The figure shows three views and two pictorial views of one solid part (mm, origin at its lowest corner). Answer the questions. A direction names the side the tool comes from. Give positions to 0.01 mm unless a question says otherwise; leave off trailing zeros. Write each loop counter-clockwise with the first axis right and the second up, starting at its lowest first coordinate (ties: lowest second). Pieces come first, ordered by that corner, then holes. Notation, with made-up numbers: (-16, 0.25) -> (18, 0.25) arc R9 ccw to (18, 5.25) -> close; hole circle Ø2 at (-12, 35). An arc over 180 degrees is marked (long way). Write each question's results on one line, items separated by ' | '. Start each with the question number.
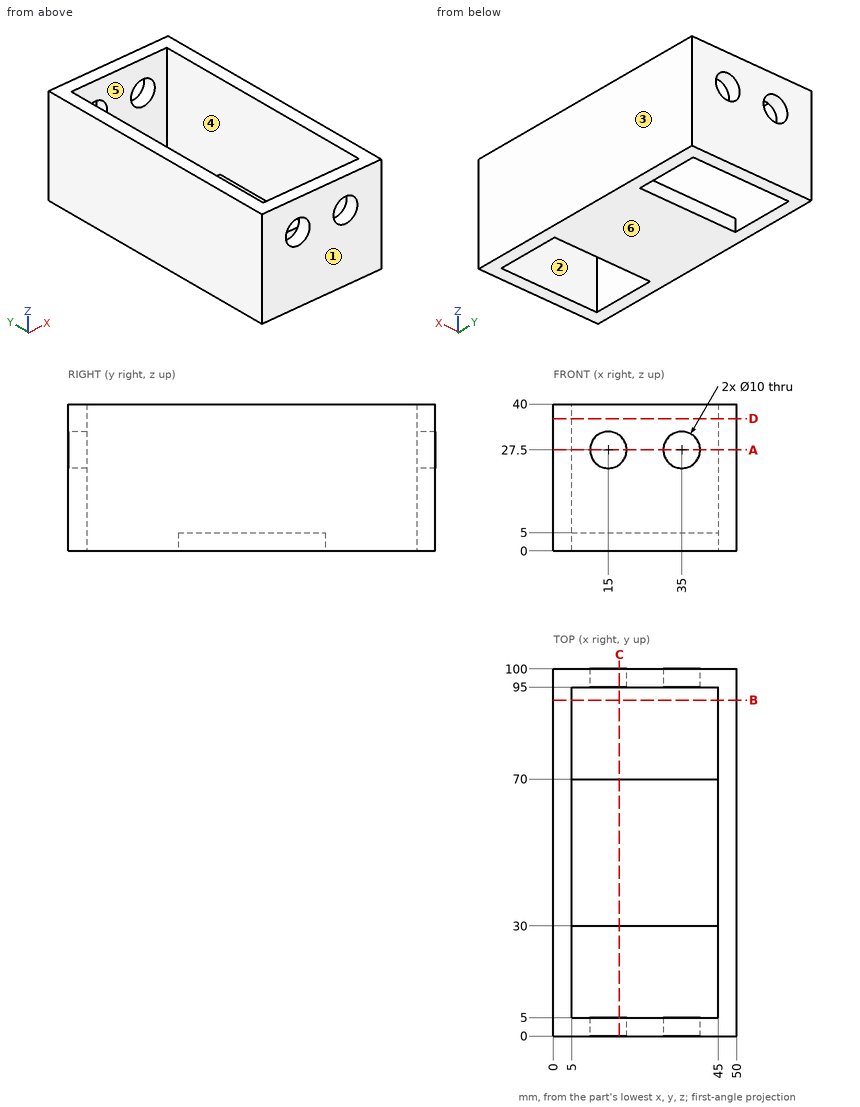
1. Consider probe 1 along Y at (x, z) = (17, 38.5); probe 2 along Z at (x, y) = (15, 97.7); probe 3 along X at (y, z) = (36, 9.5). Determine where each line is inside the solid, lowest interval first. Write a range as [from, to].
2. The mould has two halves that part along Y. Classify the marked faces 1, 2 and 3: pulls with the +Y half, pulls with the -Y half, needs draft (parallel to the pull), parting line crosses it, or undercut.
3. Section B-B (y = 91.5) is taken. Write down the section's boundary in (x, z), then the cut area to 3 significant figures.
4. Section A-A (z = 27.5) is taken. Write down the section's boundary in (x, y).
5. A tool of negligible diameter and unlimited length cuts with its end or side. For the marked faces 4, 5 and 6, from which of +Z, -Z, +X, -X, +Y, -Y can it reach the whole face along a straight path? Write none if from no direction.
6. Section D-D (z = 36) is taken. Write down the section's boundary in (x, y).
7. Section C-C (x = 18) is taken. Write down the section's boundary in (y, z), then the cut area to 3 significant figures.
8. Each of these flat-tipped pins is pushed along its axis until it touches: pin 1 Ø9 at (x, z) = (15, 27.5) entering from +Y; pin 2 Ø20 at (x, y) = (24.5, 46) entering from +Z. Where does it stop, or does it pass through?
Results:
1) probe 1: y = [0, 5], [95, 100] | probe 2: z = [0, 22.5], [32.5, 40] | probe 3: x = [0, 5], [45, 50]
2) face 1: pulls with the -Y half | face 2: undercut | face 3: needs draft
3) outline: (0, 0) -> (5, 0) -> (5, 40) -> (0, 40) -> close; (45, 0) -> (50, 0) -> (50, 40) -> (45, 40) -> close | area: 400 mm²
4) outline: (0, 0) -> (10, 0) -> (10, 5) -> (5, 5) -> (5, 95) -> (10, 95) -> (10, 100) -> (0, 100) -> close; (20, 0) -> (30, 0) -> (30, 5) -> (20, 5) -> close; (20, 95) -> (30, 95) -> (30, 100) -> (20, 100) -> close; (40, 0) -> (50, 0) -> (50, 100) -> (40, 100) -> (40, 95) -> (45, 95) -> (45, 5) -> (40, 5) -> close
5) face 4: +Z | face 5: +Z, -Z | face 6: -Z, +X, -X, +Y, -Y
6) outline: (0, 0) -> (50, 0) -> (50, 100) -> (0, 100) -> close; hole (5, 5) -> (45, 5) -> (45, 95) -> (5, 95) -> close
7) outline: (0, 0) -> (5, 0) -> (5, 23.5) -> (0, 23.5) -> close; (0, 31.5) -> (5, 31.5) -> (5, 40) -> (0, 40) -> close; (30, 0) -> (70, 0) -> (70, 5) -> (30, 5) -> close; (95, 0) -> (100, 0) -> (100, 23.5) -> (95, 23.5) -> close; (95, 31.5) -> (100, 31.5) -> (100, 40) -> (95, 40) -> close | area: 520 mm²
8) pin 1: passes through | pin 2: stops at z = 5
